Geometry: final body of the model. Coordinates: model frame, mm. Face numbers are marked on the shaded views. A direction names the side the tool comes from. Give positions to 0.01 mm unless a question says otherwise; leave off trailing zeros. Loops run counter-clockwise (first coordinate to the right, second up) from the corner with the lowest first, then second, coordinate; pieces in that order, holes last. Notation, with made-up numbers: (65, 37.25) - (119, 37.25) arc R15 cw to (119, 46.25) - close; hole circle Ø7 at (-38, 58.25). An arc over 180 degrees is marked (long way). Answer in a Markdown table with one row per item.
from build123d import *

# Parameters (mm, degrees)
SKETCH1_R           = 5
SKETCH1_R_2         = 3
BOSS_EXTRUDE1_DEPTH = 3.5
BOSS_EXTRUDE2_DEPTH = 29.918114598
CUT_EXTRUDE1_START  = -3.5
CUT_EXTRUDE1_DEPTH  = 28.5


with BuildPart() as part:
    # Sketch1 → Boss-Extrude1 (new body)
    # profile 1 of 5: a face of its own
    with BuildSketch(Plane(origin=(0, 0, 0), x_dir=(1, 0, 0), z_dir=(0, 1, 0))):
        with BuildLine():
            Line((-18.594331138, 14.849183308), (-28.753774302, 3.302904553))
            ThreePointArc((-28.753774302, 3.302904553), (-23.234903899, 4.678080349), (-20, 0))
            ThreePointArc((-20, 0), (-23.086582838, -4.619397663), (-28.535533906, -3.535533906))
            Line((-28.535533906, -3.535533906), (-3.535533906, -28.535533906))
            ThreePointArc((-3.535533906, -28.535533906), (-1.913417162, -20.380602337), (5, -25))
            ThreePointArc((5, -25), (4.619397663, -26.913417162), (3.535533906, -28.535533906))
            Line((3.535533906, -28.535533906), (28.535533906, -3.535533906))
            ThreePointArc((28.535533906, -3.535533906), (20.002544279, 0.159487685), (28.753774302, 3.302904553))
            Line((28.753774302, 3.302904553), (18.594331138, 14.849183308))
            Line((18.594331138, 14.849183308), (-18.594331138, 14.849183308))
        make_face()
    # profile 2 of 5: a face of its own
    with BuildSketch(Plane(origin=(0, 0, 0), x_dir=(1, 0, 0), z_dir=(0, 1, 0))):
        with Locations((0, -25)):
            Circle(SKETCH1_R)
        with Locations(Location((0, -25, 0), (0, 0, 270))):
            Circle(SKETCH1_R_2, mode=Mode.SUBTRACT)
    # profile 3 of 5: a face of its own
    with BuildSketch(Plane(origin=(0, 0, 0), x_dir=(1, 0, 0), z_dir=(0, 1, 0))):
        with Locations((-25, 0)):
            Circle(SKETCH1_R)
        with Locations(Location((-25, 0, 0), (0, 0, 270))):
            Circle(SKETCH1_R_2, mode=Mode.SUBTRACT)
    # profile 4 of 5: a face of its own
    with BuildSketch(Plane(origin=(0, 0, 0), x_dir=(1, 0, 0), z_dir=(0, 1, 0))):
        with Locations((25, 0)):
            Circle(SKETCH1_R)
        with Locations(Location((25, 0, 0), (0, 0, 270))):
            Circle(SKETCH1_R_2, mode=Mode.SUBTRACT)
    # profile 5 of 5: a face of its own
    with BuildSketch(Plane(origin=(0, 0, 0), x_dir=(1, 0, 0), z_dir=(0, 1, 0))):
        Polygon((0, 35.98177169), (-18.594331138, 14.849183308), (18.594331138, 14.849183308), align=None)
    extrude(amount=BOSS_EXTRUDE1_DEPTH)

    # Sketch1_3 → Boss-Extrude2 (add)
    with BuildSketch(Plane(origin=(0, 0, 0), x_dir=(1, 0, 0), z_dir=(0, 1, 0))):
        Polygon((0, 35.98177169), (-18.594331138, 14.849183308), (18.594331138, 14.849183308), align=None)
    extrude(amount=BOSS_EXTRUDE2_DEPTH)

    # Sketch3 → Cut-Extrude1 (cut)
    with BuildSketch(Plane(origin=(0, 29.918114598, 0), x_dir=(1, 0, 0), z_dir=(0, 1, 0)).offset(CUT_EXTRUDE1_START)):
        Polygon((-11.958686143, 17.849183308), (11.958686143, 17.849183308), (0, 31.440314389), align=None)
    extrude(amount=-CUT_EXTRUDE1_DEPTH, mode=Mode.SUBTRACT)


solid = part.part
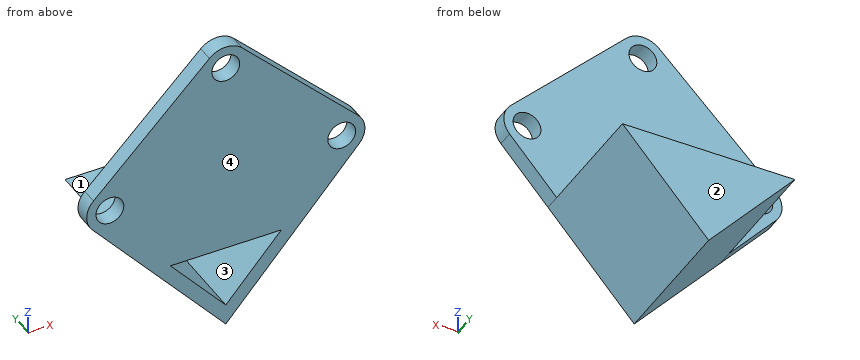
Q1. Material intervals for line 1 along Y through (x, z) = (8, -12.5); line 2 along X through (y, z) = (1.7, 25); line 3 along Y through (x, z) = (3, -27.5), sorted ascending.
Check values:
| item | result |
|---|---|
| line 1 | 0 to 3.5 |
| line 2 | -7.07 to -3, 3 to 7.07 |
| line 3 | 26.42 to 29.92 |
Q2. Cut plane D-D (x = -25). Output: boundary loops of the cut face in (y, z), and give its area (3 significant figures).
Check values:
| item | result |
|---|---|
| outline | (0, -7.57) - (3.5, -7.57) - (3.5, -3) - (0, -3) - close; (0, 3) - (3.5, 3) - (3.5, 7.07) - (0, 7.07) - close |
| area | 30.2 mm² |
Q3. First-contact query: pin 1 (1.5 mm diameter, centred on y = 6.5, z = -24.5, fed in from +X); pin 2 (3 mm diameter, centred on x = 13.5, y = 26, fed in from +Z); pin 3 (4 mm diameter, centred on x = -8.5, y = 4.5, fed in from +Z). Flat tips, straight axial feed; report the tip coordinate or a pass-through.
Check values:
| item | result |
|---|---|
| pin 1 | x = 10.76 |
| pin 2 | z = -14.85 |
| pin 3 | z = 25.3 |
Q4. Cut plane A-A (z = 0). Output: boundary loops of the cut face in (x, y).
Check values:
| item | result |
|---|---|
| outline | (-30, 0) - (-28, 0) - (-28, 3.5) - (-30, 3.5) - close; (-22, 0) - (22, 0) - (22, 3.5) - (-22, 3.5) - close; (28, 0) - (30, 0) - (30, 3.5) - (28, 3.5) - close |
Q5. Reachability of the marked faces 1 and 2 from +Z, -Z, +X, -X, +Y, -Y: full face, straight path, thin tool, end or side. Return the list, or none.
Check values:
| item | result |
|---|---|
| face 1 | +Z, +X, -X, +Y |
| face 2 | +Z, -Z, +X, -X, +Y |
Q6. Draft query along X for the marked faces 3 and 4. Return one class per face: pulls with the +X half, pulls with the -X half, needs draft (parallel to the pull), parting line crosses it, or undercut.
Check values:
| item | result |
|---|---|
| face 3 | undercut |
| face 4 | needs draft |
Q7. Cut plane B-B (y = 24). Output: boundary loops of the cut face in (x, z), and give its area (3 significant figures).
Check values:
| item | result |
|---|---|
| outline | (-18.59, -14.85) - (0, -35.98) - (18.59, -14.85) - close; hole (-11.96, -17.85) - (0, -31.44) - (11.96, -17.85) - close |
| area | 230 mm² |
Q8. Cut plane C-C (z = 25). Output: boundary loops of the cut face in (x, y), and give its area (3 significant figures).
Check values:
| item | result |
|---|---|
| outline | (-7.07, 0) - (-3, 0) - (-3, 3.5) - (-7.07, 3.5) - close; (3, 0) - (7.07, 0) - (7.07, 3.5) - (3, 3.5) - close |
| area | 28.5 mm² |
